from build123d import *

# Parameters (mm, degrees)
SKETCH2_R               = 21.36
BOSS_EXTRUDE1_DEPTH     = 300
SHELL1_T                = -4
SKETCH3_W               = 54.462291246
SKETCH3_H               = 357.024978236
CUT_EXTRUDE1_DEPTH      = 302.516996536
CUT_EXTRUDE1_DEPTH_BACK = 302.516996536


with BuildPart() as part:
    # Sketch2 → Boss-Extrude1 (new body)
    with BuildSketch(Plane(origin=(0, 0, 0), x_dir=(1, 0, 0), z_dir=(0, 1, 0))):
        with Locations(Location((0, 0, 0), (0, 0, 270))):
            Circle(SKETCH2_R)
    extrude(amount=BOSS_EXTRUDE1_DEPTH)

    # Shell1
    shell1_openings = [part.faces().sort_by_distance(p)[0] for p in [
        (0, 300, 0),
        (0, 0, 0),
    ]]
    offset(amount=SHELL1_T, openings=shell1_openings, kind=Kind.INTERSECTION)

    # Sketch3 → Cut-Extrude1 (cut, two sides)
    with BuildSketch(Plane(origin=(0, 0, 0), x_dir=(0, 0, -1), z_dir=(1, 0, 0))) as cut_extrude1_sk:
        with Locations((27.231145623, 138.076503498)):
            Rectangle(SKETCH3_W, SKETCH3_H)
    extrude(amount=CUT_EXTRUDE1_DEPTH, mode=Mode.SUBTRACT)
    extrude(cut_extrude1_sk.sketch, amount=-CUT_EXTRUDE1_DEPTH_BACK, mode=Mode.SUBTRACT)


solid = part.part
Geometry check sheet. Reference: the model listing, model coordinates, mm. Give positions to 0.01 mm unless a question says otherwise; leave off trailing zeros. Write each loop counter-clockwise with the first axis right and the second up, starting at its lowest first coordinate (ties: lowest second). Pieces come first, ordered by that corner, then holes.
1) Go/stop test with flat-tipped pins: pin 1 Ø5 at (x, y) = (15, 97) entering from +Z; pin 2 Ø8 at (y, z) = (49, 5.5) entering from +X; pin 3 Ø6 at (x, y) = (8, 36.5) entering from -Z; pin 4 Ø12 at (x, z) = (1.5, 14) entering from -Y. Record where each tip stops, or that it passes through.
Values follow:
pin 1: stops at z = 17.32
pin 2: stops at x = 21.31
pin 3: stops at z = 13.43
pin 4: stops at y = 0
2) Release check for a two-part mould opening along X. For faces 1 (the face through (-0.47, 147.9, 21.355)), 2 (the face through (-0.382, 147.9, 17.356)), 3 (the face through (2, 0, 18)) record: released by +X, released by -X, zero draft, split by the parting line, or undercut.
Values follow:
face 1: split by the parting line
face 2: undercut
face 3: zero draft
3) Cross-section at B-B (y = 262). Record the boundary of the cut face in (x, z), plus the area to 3 significant figures.
Values follow:
outline: (-21.36, 0) - (-17.36, 0) arc R17.36 cw to (17.36, 0) - (21.36, 0) arc R21.36 ccw to start
area: 243 mm2
4) Cross-section at C-C (x = 0). Record the boundary of the cut face in (y, z).
Values follow:
outline: (0, 17.36) - (300, 17.36) - (300, 21.36) - (0, 21.36) - close
5) Thickness scan on line 1 (X direction, y = 166.5, z = 12.5); line 2 (Z direction, x = -1, y = 27.5); line 3 (X direction, y = 35, z = 14.75). Record the ranges inside material, lowest first.
Values follow:
line 1: x = -17.32 to -12.05, 12.05 to 17.32
line 2: z = 17.33 to 21.34
line 3: x = -15.45 to -9.15, 9.15 to 15.45
6) Cross-section at D-D (z = 14.5). Record the boundary of the cut face in (x, y).
Values follow:
outline: (-15.68, 0) - (-9.55, 0) - (-9.55, 300) - (-15.68, 300) - close; (9.55, 0) - (15.68, 0) - (15.68, 300) - (9.55, 300) - close
7) Cross-section at A-A (z = 3.75). Record the boundary of the cut face in (x, y).
Values follow:
outline: (-21.03, 0) - (-16.95, 0) - (-16.95, 300) - (-21.03, 300) - close; (16.95, 0) - (21.03, 0) - (21.03, 300) - (16.95, 300) - close
